```python
from build123d import *

# Parameters (mm, degrees)
SKETCH2_R                = 7.62
BOSS_EXTRUDE1_DEPTH      = 34.29
SKETCH3_R                = 7.62
BOSS_EXTRUDE2_DEPTH      = 17.145
BOSS_EXTRUDE2_DEPTH_BACK = 17.145
FILLET1_R                = 1.27
SCALE1_SCALE             = 2


with BuildPart() as part:
    # Sketch2 → Boss-Extrude1 (new body)
    with BuildSketch(Plane.XY):
        Circle(SKETCH2_R)
    extrude(amount=BOSS_EXTRUDE1_DEPTH)

    # Sketch3 → Boss-Extrude2 (add, two sides)
    with BuildSketch(Plane(origin=(0, 0, 0), x_dir=(0, 0, -1), z_dir=(1, 0, 0))) as boss_extrude2_sk:
        with Locations((-17.145, 0)):
            Circle(SKETCH3_R)
    extrude(amount=BOSS_EXTRUDE2_DEPTH)
    extrude(boss_extrude2_sk.sketch, amount=-BOSS_EXTRUDE2_DEPTH_BACK)

    # Fillet1
    fillet1_edges = [part.edges().sort_by_distance(p)[0] for p in [
        (-7.62, 0, 0),
        (-7.62, 0, 34.29),
        (-17.145, 0, 24.765),
        (17.145, 0, 24.765),
    ]]
    fillet(fillet1_edges, radius=FILLET1_R)


with BuildPart() as part_1:
    # Scale1: scaled about (0, 0, 17.145)
    add(part.part.scale(SCALE1_SCALE).moved(Location((0, 0, -17.145))))


solid = part_1.part
```
Geometry: final body of the model. Coordinates: model frame, mm. A direction names the side the tool comes from. Round coordinates to 2 decimals unless told otherwise and drop trailing zeros. Write each loop counter-clockwise with the first axis right and the second up, starting at its lowest first coordinate (ties: lowest second). Pieces come first, ordered by that corner, then holes. Notation, with made-up numbers: (68, 22.5) -> (108, 22.5) arc R23 cw to (108, 51.5) -> close; hole circle Ø7 at (-26, 79.25). An arc over 180 degrees is marked (long way). Return JSON: item names as keys, results as strings.
Q1. Set-up query: faces 1 (the cylindrical face through (-11.23, 10.3, -2.48)), 2 (the cylindrical face through (-15.225, 0.67, 36.326)), 3 (the cylindrical face through (-19.18, 0.67, 32.37)), 4 (the cylindrical face through (19.18, 0.67, 32.37)). Return all of +Z, -Z, +X, -X, +Y, -Y with unobstructed straight access to the full face (end or side cutting, diameter ignored); none if empty.
From the geometry:
{"face 1": "-Z", "face 2": "+Z", "face 3": "-X", "face 4": "+X"}
Q2. First-contact query: pin 1 Ø1.5 at (y, z) = (-3, 1) entering from +X; pin 2 Ø3 at (x, y) = (-13, 5.5) entering from +Z (3 decimals); pin 3 Ø2 at (x, y) = (26, 8.5) entering from -Z; pin 4 Ø4 at (y, z) = (7.5, 33) entering from -X. Flat tips, straight axial feed; report the tip coordinate or a pass-through.
From the geometry:
{"pin 1": "x = 15.07", "pin 2": "z = 51.435", "pin 3": "z = 3.88", "pin 4": "x = -14.21"}
Q3. Ray query, line 1 (Y direction, x = -7.5, z = 31.5); line 2 (Y direction, x = 11, z = 8); line 3 (X direction, y = 9, z = 31). Return the intervals inside material, ascending.
From the geometry:
{"line 1": "-13.27 to 13.27", "line 2": "-12.19 to 12.19", "line 3": "-12.3 to 12.3"}
Q4. Section A-A on y = 0. Return the cut outline in (x, z) (3 decimals), and give its area (3 significant figures).
From the geometry:
{"outline": "(-34.29, 4.445) arc R2.54 ccw to (-31.75, 1.905) -> (-15.24, 1.905) -> (-15.24, -14.605) arc R2.54 ccw to (-12.7, -17.145) -> (12.7, -17.145) arc R2.54 ccw to (15.24, -14.605) -> (15.24, 1.905) -> (31.75, 1.905) arc R2.54 ccw to (34.29, 4.445) -> (34.29, 29.845) arc R2.54 ccw to (31.75, 32.385) -> (15.24, 32.385) -> (15.24, 48.895) arc R2.54 ccw to (12.7, 51.435) -> (-12.7, 51.435) arc R2.54 ccw to (-15.24, 48.895) -> (-15.24, 32.385) -> (-31.75, 32.385) arc R2.54 ccw to (-34.29, 29.845) -> close", "area": "3,240 mm2"}
Q5. Section B-B on x = 29. Return the cut outline in (y, z) (3 decimals), and give its area (3 significant figures).
From the geometry:
{"outline": "circle Ø30.48 at (0, 17.145)", "area": "730 mm2"}
